Work out the finished part from the listing and answer in its coordinate system (mm). Coordinates: 2 decimals unless noted, no trailing zeros. Order: outer loops, then holes, each group sorted by start corner. A loop starts at its lowest first (then second) coordinate and runs counter-clockwise, first axis right, second up. Notation, with made-up numbers: (-36, -1) - (-16, -1) arc R9 cw to (-16, 9) - close; hole circle Ø10 at (19.25, 86.25). An arc over 180 degrees is marked (long way). Answer as a JSON object with one key per item and string values. Group by question number.
1) Section D-D (x = 173) is taken. Give the vertices of the cut face in (y, z).
2) Find the intervals of material crossed by line 1 along Y through (x, z) = (112.5, 1.5); line 2 along Y through (x, z) = (83, 2); line 3 along X through (y, z) = (28, 2.45), in increasing order.
3) Section B-B (y = 0) is taken. Give the vertices of the cut face in (x, z), plus the area to 3 significant figures.
4) Section C-C (y = -15) is taken. Give the vertices of the cut face in (x, z).
5) Each of these flat-tipped pins is pushed along its axis until it touches: P1, Ø1.8, axis at x = 44.22, y = 21.98, coming from the -Z side; P2, Ø5, axis at x = 149.22, y = -9.26, coming from the -Z side; P3, Ø1.5, axis at y = 9.5, z = 2, coming from the +X side; P4, Ø1.5, axis at y = -24.5, z = 0.5, coming from the -X side. Where does it stop, or does it pass through?
6) Section A-A (x = 76) is taken. Give the vertices of the cut face in (y, z).
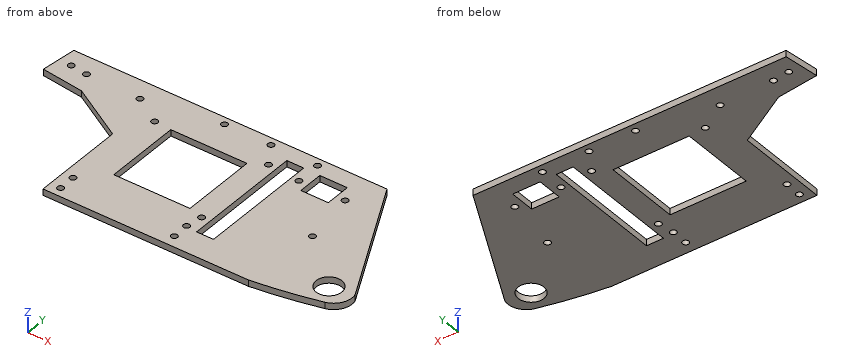
from build123d import *

# Parameters (mm, degrees)
EXTRUDE_1_DEPTH     = 3
CUT_EXTRUDE_1_REACH = 5
SKETCH_2_R          = 6.1
SKETCH_2_W          = 36
SKETCH_2_H          = 36
MM_CLEARANCE_1_D    = 3
MM_CLEARANCE_4_D    = 3
CUT_EXTRUDE_2_REACH = 5
SKETCH_18_R         = 1.5
MM_CLEARANCE_6_D    = 3
CUT_EXTRUDE_3_REACH = 5
SKETCH_21_W         = 13
SKETCH_21_H         = 12
MM_CLEARANCE_7_D    = 3
MM_CLEARANCE_10_D   = 3


with BuildPart() as part:
    # 草图1 → 凸台-拉伸1 (new body)
    with BuildSketch(Plane.XY):
        with BuildLine():
            Line((30.367519571, 31.798067496), (153.728402084, 31.798067496))
            Line((153.728402084, 31.798067496), (184.602796718, -29.595613307))
            ThreePointArc((184.602796718, -29.595613307), (183.670445617, -36.224755467), (178.320075375, -40.248229416))
            ThreePointArc((178.320075375, -40.248229416), (162.522923857, -43.753908616), (146.527707017, -46.201932504))
            Line((146.527707017, -46.201932504), (49.449368769, -46.201932504))
            Line((49.449368769, -46.201932504), (49.449368769, -2.201932504))
            Line((49.449368769, -2.201932504), (23.468606655, 12.798067496))
            Line((23.468606655, 12.798067496), (3.617683623, 15.235454364))
            Line((3.617683623, 15.235454364), (5.651316803, 31.798067496))
            Line((5.651316803, 31.798067496), (5.659575981, 31.798067496))
            Line((5.659575981, 31.798067496), (30.367519571, 31.798067496))
        make_face()
    extrude(amount=EXTRUDE_1_DEPTH)

    # 草图2 → 切除-拉伸1 (cut, up to next)
    with BuildSketch(Plane.XY.offset(3), mode=Mode.PRIVATE) as cut_extrude_1_sk1:
        with Locations((173.449368769, -31.201932504)):
            Circle(SKETCH_2_R)
    cut_extrude_1_tool1 = extrude(cut_extrude_1_sk1.sketch, amount=-CUT_EXTRUDE_1_REACH, mode=Mode.PRIVATE) & part.part
    add(cut_extrude_1_tool1.solids().sort_by_distance((173.449369, -31.201933, 3))[0], mode=Mode.SUBTRACT)
    # 草图2 → 切除-拉伸1 (cut, up to next)
    with BuildSketch(Plane.XY.offset(3), mode=Mode.PRIVATE) as cut_extrude_1_sk2:
        with Locations((83.439887491, -4.827295438)):
            Rectangle(SKETCH_2_W, SKETCH_2_H)
    cut_extrude_1_tool2 = extrude(cut_extrude_1_sk2.sketch, amount=-CUT_EXTRUDE_1_REACH, mode=Mode.PRIVATE) & part.part
    add(cut_extrude_1_tool2.solids().sort_by_distance((83.439887, -4.827295, 3))[0], mode=Mode.SUBTRACT)
    # 草图2 → 切除-拉伸1 (cut, up to next)
    with BuildSketch(Plane.XY.offset(3), mode=Mode.PRIVATE) as cut_extrude_1_sk3:
        Polygon((112.439887491, -4.827295438), (112.439887491, -33.327295438), (120.439887491, -33.327295438), (120.439887491, 23.672704562), (112.439887491, 23.672704562), align=None)
    cut_extrude_1_tool3 = extrude(cut_extrude_1_sk3.sketch, amount=-CUT_EXTRUDE_1_REACH, mode=Mode.PRIVATE) & part.part
    add(cut_extrude_1_tool3.solids().sort_by_distance((116.439887, -4.827295, 3))[0], mode=Mode.SUBTRACT)

    # 大小mm Clearance 暗销孔1 (through all)
    with Locations(Plane(origin=(141.673702765, 151.858231724, 3), x_dir=(-0.99978014, -0.020968354, 0), z_dir=(0, 0, 1))):
        with Locations((20.591231353, 123.39816829), (42.591231353, 122.936763059), (64.581557509, 122.475560716)):
            Hole(MM_CLEARANCE_1_D / 2)

    # 大小mm Clearance 暗销孔4 (through all)
    with Locations(Plane(origin=(141.673702765, 151.858231724, 3), x_dir=(-0.99978014, -0.020968354, 0), z_dir=(0, 0, 1))):
        with Locations((20.608818994, 135.452556109), (-0.900285243, 135.452556109)):
            Hole(MM_CLEARANCE_4_D / 2)

    # 草图18 → 切除-拉伸2 (cut, up to next)
    with BuildSketch(Plane.XY.offset(3), mode=Mode.PRIVATE) as cut_extrude_2_sk1:
        with Locations((149.222841692, -9.258973797)):
            Circle(SKETCH_18_R)
    cut_extrude_2_tool1 = extrude(cut_extrude_2_sk1.sketch, amount=-CUT_EXTRUDE_2_REACH, mode=Mode.PRIVATE) & part.part
    add(cut_extrude_2_tool1.solids().sort_by_distance((149.222842, -9.258974, 3))[0], mode=Mode.SUBTRACT)

    # 大小mm Clearance 暗销孔6 (through all)
    with Locations(Plane(origin=(141.673702765, 151.858231724, 3), x_dir=(-0.99978014, -0.020968354, 0), z_dir=(0, 0, 1))):
        with Locations((36.045400202, 133.709111751), (36.930668673, 175.919093371)):
            Hole(MM_CLEARANCE_6_D / 2)

    # 草图21 → 切除-拉伸3 (cut, up to next)
    with BuildSketch(Plane.XY.offset(3), mode=Mode.PRIVATE) as cut_extrude_3_sk1:
        with Locations((134.661819591, 17.503323217)):
            Rectangle(SKETCH_21_W, SKETCH_21_H)
    cut_extrude_3_tool1 = extrude(cut_extrude_3_sk1.sketch, amount=-CUT_EXTRUDE_3_REACH, mode=Mode.PRIVATE) & part.part
    add(cut_extrude_3_tool1.solids().sort_by_distance((134.66182, 17.503323, 3))[0], mode=Mode.SUBTRACT)

    # 大小mm Clearance 暗销孔7 (through all)
    with Locations(Plane(origin=(143.321207743, 150.868006211, 3), x_dir=(-0.99975237, -0.022253058, 0), z_dir=(0, 0, 1))):
        with Locations((88.938953066, 135.227377046), (101.942467158, 126.647536361), (127.53759353, 125.598807912), (135.454300746, 124.4473971)):
            Hole(MM_CLEARANCE_7_D / 2)

    # 大小mm Clearance 暗销孔10 (through all)
    with Locations(Plane(origin=(143.321207743, 150.868006211, 3), x_dir=(-0.99975237, -0.022253058, 0), z_dir=(0, 0, 1))):
        with Locations((93.161367469, 190.578219389), (93.161367469, 182.547127137), (40.245392963, 190.578219389), (40.245392963, 182.547127137)):
            Hole(MM_CLEARANCE_10_D / 2)


solid = part.part
Report:
{
 "1": {"outline": "(-41.55, 0) - (-37.29, 0) - (-37.29, 3) - (-41.55, 3) - close; (-25.12, 0) - (-6.52, 0) - (-6.52, 3) - (-25.12, 3) - close"},
 "2": {"line 1": "y = -46.2 to -33.33, 23.67 to 31.8", "line 2": "y = -46.2 to -22.83, 13.17 to 31.8", "line 3": "x = 5.18 to 78.18, 81.17 to 100.17, 103.17 to 122.18, 125.17 to 155.64"},
 "3": {"outline": "(45.64, 0) - (65.44, 0) - (65.44, 3) - (45.64, 3) - close; (101.44, 0) - (112.44, 0) - (112.44, 3) - (101.44, 3) - close; (120.44, 0) - (169.72, 0) - (169.72, 3) - (120.44, 3) - close", "area": "240 mm²"},
 "4": {"outline": "(49.45, 0) - (65.44, 0) - (65.44, 3) - (49.45, 3) - close; (101.44, 0) - (112.44, 0) - (112.44, 3) - (101.44, 3) - close; (120.44, 0) - (177.26, 0) - (177.26, 3) - (120.44, 3) - close"},
 "5": {"P1": "passes through", "P2": "stops at z = 0", "P3": "stops at x = 165.32", "P4": "stops at x = 49.45"},
 "6": {"outline": "(-46.2, 0) - (-22.83, 0) - (-22.83, 3) - (-46.2, 3) - close; (13.17, 0) - (31.8, 0) - (31.8, 3) - (13.17, 3) - close"}
}
